from build123d import *

# Parameters (mm, degrees)
F0_R          = 13.8
F1_DEPTH      = 16
F1_DEPTH_BACK = 6
F2_R          = 13.8
F3_DEPTH      = 2


with BuildPart() as f1:
    # F0 (on Top) → F1 (new body, two sides)
    with BuildSketch(Plane.XY) as f1_sk:
        Circle(F0_R)
        with BuildLine():
            Line((-1.270171, 8.7), (0, 8.7))
            Line((0, 8.7), (1.270171, 8.7))
            ThreePointArc((1.270171, 8.7), (1.770171, 8.833975), (2.136196, 9.2))
            Line((2.136196, 9.2), (3.11843, 10.901279))
            ThreePointArc((3.11843, 10.901279), (3.725636, 11.367205), (4.484456, 11.267305))
            Line((4.484456, 11.267305), (6, 10.392305))
            Line((6, 10.392305), (7.515544, 9.517305))
            ThreePointArc((7.515544, 9.517305), (7.98147, 8.910098), (7.88157, 8.151279))
            Line((7.88157, 8.151279), (6.899336, 6.45))
            ThreePointArc((6.899336, 6.45), (6.765361, 5.95), (6.899336, 5.45))
            Line((6.899336, 5.45), (7.534421, 4.35))
            Line((7.534421, 4.35), (8.169506, 3.25))
            ThreePointArc((8.169506, 3.25), (8.535532, 2.883975), (9.035532, 2.75))
            Line((9.035532, 2.75), (11, 2.75))
            ThreePointArc((11, 2.75), (11.707107, 2.457107), (12, 1.75))
            Line((12, 1.75), (12, 0))
            Line((12, 0), (12, -1.75))
            ThreePointArc((12, -1.75), (11.707107, -2.457107), (11, -2.75))
            Line((11, -2.75), (9.035532, -2.75))
            ThreePointArc((9.035532, -2.75), (8.535532, -2.883975), (8.169506, -3.25))
            Line((8.169506, -3.25), (7.534421, -4.35))
            Line((7.534421, -4.35), (6.899336, -5.45))
            ThreePointArc((6.899336, -5.45), (6.765361, -5.95), (6.899336, -6.45))
            Line((6.899336, -6.45), (7.88157, -8.151279))
            ThreePointArc((7.88157, -8.151279), (7.98147, -8.910098), (7.515544, -9.517305))
            Line((7.515544, -9.517305), (6, -10.392305))
            Line((6, -10.392305), (4.484456, -11.267305))
            ThreePointArc((4.484456, -11.267305), (3.725636, -11.367205), (3.11843, -10.901279))
            Line((3.11843, -10.901279), (2.136196, -9.2))
            ThreePointArc((2.136196, -9.2), (1.770171, -8.833975), (1.270171, -8.7))
            Line((1.270171, -8.7), (0, -8.7))
            Line((0, -8.7), (-1.270171, -8.7))
            ThreePointArc((-1.270171, -8.7), (-1.770171, -8.833975), (-2.136196, -9.2))
            Line((-2.136196, -9.2), (-3.11843, -10.901279))
            ThreePointArc((-3.11843, -10.901279), (-3.725636, -11.367205), (-4.484456, -11.267305))
            Line((-4.484456, -11.267305), (-6, -10.392305))
            Line((-6, -10.392305), (-7.515544, -9.517305))
            ThreePointArc((-7.515544, -9.517305), (-7.98147, -8.910098), (-7.88157, -8.151279))
            Line((-7.88157, -8.151279), (-6.899336, -6.45))
            ThreePointArc((-6.899336, -6.45), (-6.765361, -5.95), (-6.899336, -5.45))
            Line((-6.899336, -5.45), (-7.534421, -4.35))
            Line((-7.534421, -4.35), (-8.169506, -3.25))
            ThreePointArc((-8.169506, -3.25), (-8.535532, -2.883975), (-9.035532, -2.75))
            Line((-9.035532, -2.75), (-11, -2.75))
            ThreePointArc((-11, -2.75), (-11.707107, -2.457107), (-12, -1.75))
            Line((-12, -1.75), (-12, 0))
            Line((-12, 0), (-12, 1.75))
            ThreePointArc((-12, 1.75), (-11.707107, 2.457107), (-11, 2.75))
            Line((-11, 2.75), (-9.035532, 2.75))
            ThreePointArc((-9.035532, 2.75), (-8.535532, 2.883975), (-8.169506, 3.25))
            Line((-8.169506, 3.25), (-7.534421, 4.35))
            Line((-7.534421, 4.35), (-6.899336, 5.45))
            ThreePointArc((-6.899336, 5.45), (-6.765361, 5.95), (-6.899336, 6.45))
            Line((-6.899336, 6.45), (-7.88157, 8.151279))
            ThreePointArc((-7.88157, 8.151279), (-7.98147, 8.910098), (-7.515544, 9.517305))
            Line((-7.515544, 9.517305), (-6, 10.392305))
            Line((-6, 10.392305), (-4.484456, 11.267305))
            ThreePointArc((-4.484456, 11.267305), (-3.725636, 11.367205), (-3.11843, 10.901279))
            Line((-3.11843, 10.901279), (-2.136196, 9.2))
            ThreePointArc((-2.136196, 9.2), (-1.770171, 8.833975), (-1.270171, 8.7))
        make_face(mode=Mode.SUBTRACT)
    extrude(amount=F1_DEPTH)
    extrude(f1_sk.sketch, amount=-F1_DEPTH_BACK)

    # F2 (on Top) → F3 (join)
    with BuildSketch(Plane.XY):
        Circle(F2_R)
    extrude(amount=-F3_DEPTH)


solid = f1.part
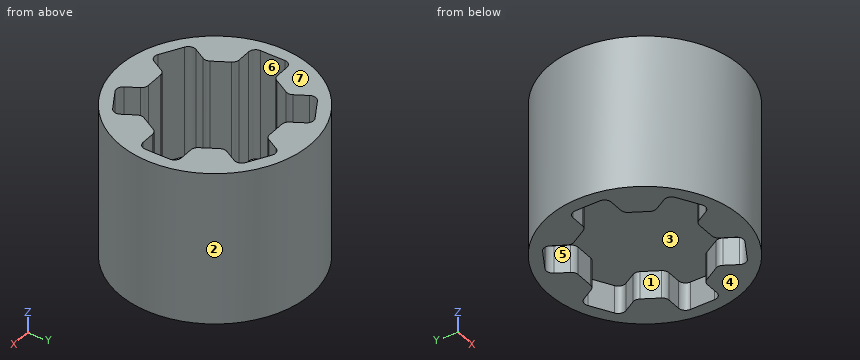
Work out the finished part from the listing and answer in its coordinate system (mm). Face numbers are marked on the shaded views. A direction names the side the tool comes from. Coordinates: 2 decimals unless noted, no trailing zeros. Write each loop counter-clockwise with the first axis right and the second up, starting at its lowest first coordinate (ties: lowest second). Pieces come first, ordered by that corner, then holes. Notation, with made-up numbers: M 82,85 L 97,85 A28 ccw 97,124 Z; hole C -28,50 d1. An arc over 180 degrees is marked long. Write item = value, one per line.
1. Straight lines are drawn through the part: line 1 (X direction, y = 9.25, z = 13); line 2 (Y direction, x = 0, z = 1); line 3 (X direction, y = -10, z = 0.75). For each, find the intervals that lie inside material, in ascending order. Write a range as from..to.
Solution:
line_1 = -10.24..-7.82, -2.17..2.17, 7.82..10.24
line_2 = -13.8..-8.7, 8.7..13.8
line_3 = -9.51..-6.68, -2.6..2.6, 6.68..9.51
2. Determine the mould class of the marked faces 1, 2, 3 and 4 for opening direction Y: released by +Y, released by -Y, zero draft, split by the parting line, or undercut.
Solution:
face_1 = undercut
face_2 = split by the parting line
face_3 = undercut
face_4 = zero draft
3. Flat-ended cylindrical pins translate along their axes: pin 1 (3 mm diameter, centred on x = 10, z = 7.5, fed in from +Y); pin 2 (5 mm diameter, centred on x = -1, y = 2, fed in from -Z); pin 3 (1.6 mm diameter, centred on x = 9.5, z = 6.5, fed in from +Y). Find the tip coordinate at first contact, or state that the pin passes through.
Solution:
pin_1 = 10.87
pin_2 = -2
pin_3 = 10.71
4. The part is cut by section B-B (y = 0). Determine the outline of the cut face in (x, z), then the cut area to 3 significant figures.
Solution:
outline = M -13.8,-6 L -12,-6 L -12,-2 L 12,-2 L 12,-6 L 13.8,-6 L 13.8,16 L 12,16 L 12,0 L -12,0 L -12,16 L -13.8,16 Z
area = 127 mm2
5. For the marked faces 5, 6 and 7, determine the directions among +Z, -Z, +X, -X, +Y, -Y from which every point of the face is accessible in a straight line to the end or side of a thin tool.
Solution:
face_5 = -Z
face_6 = +Z
face_7 = +Z, +X, -X, +Y, -Y
6. The part is cut by section A-A (x = 0). Determine the outline of the cut face in (y, z), then the cut area to 3 significant figures.
Solution:
outline = M -13.8,-6 L -8.7,-6 L -8.7,-2 L 8.7,-2 L 8.7,-6 L 13.8,-6 L 13.8,16 L 8.7,16 L 8.7,0 L -8.7,0 L -8.7,16 L -13.8,16 Z
area = 259 mm2
